Read the model definition and answer for the solid it produces. Units are mm, in the model's axes. Face numbers are marked on the shaded views. A direction names the side the tool comes from. Give positions to 0.01 mm unless a question says otherwise; leave off trailing zeros. Loops run counter-clockwise (first coordinate to the right, second up) from the corner with the lowest first, then second, coordinate; pieces in that order, holes last. Notation, with made-up numbers: (22.5, 25.25) -> (68.5, 25.25) arc R16 ccw to (68.5, 47.25) -> close; hole circle Ø5 at (-25, 10.5). An arc over 180 degrees is marked (long way). Return JSON: item names as keys, results as strings. Group by question number.
Autodesk Inventor part; units mm, degrees
ref_plane "YZ Plane" through (0, 0, 0) normal (1, 0, 0) x (0, 1, 0)
ref_plane "XZ Plane" through (0, 0, 0) normal (0, 1, 0) x (-1, 0, 0)
ref_plane "XY Plane" through (0, 0, 0) normal (0, 0, 1) x (1, 0, 0)
sketch "Sketch1" plane through (0, 0, 0) normal (0, 1, 0) x (-1, 0, 0)
  line L0 (41.275, 29.845) -> (-4.445, 29.845)
  line L1 (-4.445, 29.845) -> (-4.445, -10.795)
  line L2 (-4.445, -10.795) -> (41.275, -10.795)
  line L3 (41.275, -10.795) -> (41.275, 29.845)
  circle A0 centre (36.83, 19.05) radius 2.54
  circle A1 centre (36.83, 0) radius 2.54
  circle A2 centre (0, 0) radius 2.54
  circle A3 centre (0, 19.05) radius 2.54
  dimension "d1" = 19.05
  dimension "d2" = 36.83
  dimension "d20" = 40.64
  dimension "d21" = 45.72
  dimension "d22" = 10.795
  dimension "d23" = 4.445
  dimension "d24" = 19.05
  dimension "d25" = 10.795
  dimension "d26" = 36.83
  dimension "d27" = 4.445
  dimension "d28" = 4.445
  dimension "d31" = 5.08
  dimension "d32" = 5.08
  dimension "d33" = 5.08
  dimension "d34" = 5.08
extrude "Extrusion5" add sketch "Sketch1" along normal blind 40.64
sketch "Sketch4" plane through (0, 40.64, 0) normal (0, 1, 0) x (1, 0, 0)
  point P0 (0, 0)
  point P1 (-18.4878, -9.5896)
sketch "Sketch5" plane through (4.445, 0, 29.845) normal (1, 0, 0) x (0, 0, -1)
  line L0 (0, 40.64) -> (40.64, 0)
  line L1 (40.64, 40.64) -> (0, 0)
  circle A0 centre (20.32, 20.32) radius 7.62
  point P0 (29.845, 0)
  dimension "d38" = 15.24
extrude "Extrusion6" add sketch "Sketch5" along normal blind 40.64
sketch "Sketch6" plane through (-41.275, 0, -10.795) normal (-1, 0, 0) x (0, 0, 1)
  line L0 (0, 40.64) -> (40.64, 0)
  line L1 (40.64, 40.64) -> (0, 0)
  circle A0 centre (20.32, 20.32) radius 20.32
  point P0 (10.795, 0)
  dimension "d41" = 40.64
extrude "Extrusion7" add sketch "Sketch6" along normal blind 50.8
properties part number "P60 Gear Box"
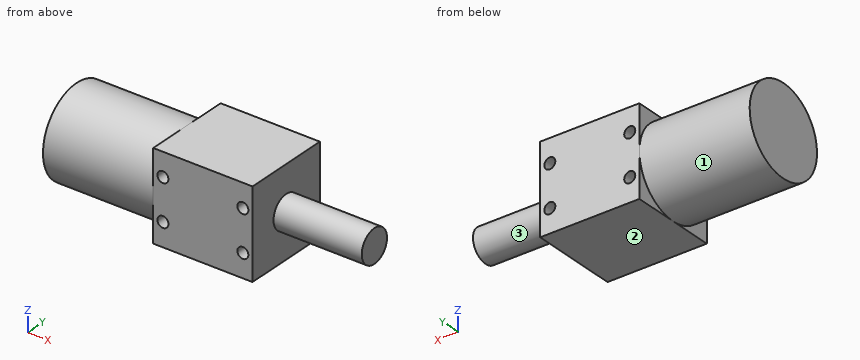
1. Section D-D on y = 23 is taken. State how many separate pieces and enclosed holes the cut face has, then the cut area to 3 significant figures.
2. Which of the six approach directions +Z, -Z, +X, -X, +Y, -Y give full straight-line access (tool end or side, diameter ignored) to the marked faces 1, 2 and 3?
3. Flat-ended cylindrical pins translate along their axes: pin 1 Ø6.5 at (x, z) = (0, 19.05) entering from +Y; pin 2 Ø3 at (x, y) = (-58, 32) entering from +Z; pin 3 Ø5 at (x, z) = (13.5, 11.5) entering from +Y; pin 4 Ø1.5 at (y, z) = (35, -3) entering from +X (3 decimals). Find the tip coordinate at first contact, or state that the pin passes through.
4. Straight lines are drawn through the part: line 1 (Z direction, x = 0, y = 17.5) (3 decimals); line 2 (X direction, y = 28, z = 19) (1 decimal); line 3 (Z direction, x = -36, y = 26) (3 decimals). For each, find the intervals that lie inside material, in ascending order. Write a range as from..to.
5. Section B-B on z = 19.05 is taken. Determine the outline of the cut face in (x, y) (3 decimals), then the cut area to 3 significant figures.
6. Section C-C on y = 33.5 is taken. Determine the outline of the cut face in (x, z) (3 decimals).
7. Section A-A on x = -36.83 is taken. Determine the outline of the cut face in (y, z) (3 decimals).
Completed:
{
 "1": {"separate pieces": "1", "enclosed holes": "4", "area": "4,400 mm²"},
 "2": {"face 1": "-X", "face 2": "-Z, +X, -X, +Y, -Y", "face 3": "+X"},
 "3": {"pin 1": "stops at y = 40.64", "pin 2": "stops at z = 27.11", "pin 3": "stops at y = 27.94", "pin 4": "stops at x = 4.445"},
 "4": {"line 1": "z = -10.795..-2.54, 2.54..16.51, 21.59..29.845", "line 2": "x = -92.1..-39.4, -34.3..-2.5, 2.5..4.4", "line 3": "z = -10.795..-2.401, 2.401..16.649, 21.451..29.845"},
 "5": {"outline": "(-92.075, 2.371) -> (-41.275, 2.371) -> (-41.275, 0) -> (-39.37, 0) -> (-39.37, 40.64) -> (-41.275, 40.64) -> (-41.275, 38.269) -> (-92.075, 38.269) -> close; (-34.29, 0) -> (-2.54, 0) -> (-2.54, 40.64) -> (-34.29, 40.64) -> close; (2.54, 0) -> (4.445, 0) -> (4.445, 40.64) -> (2.54, 40.64) -> close", "area": "3,270 mm²"},
 "6": {"outline": "(-92.075, -5.941) -> (-41.275, -5.941) -> (-41.275, -10.795) -> (4.445, -10.795) -> (4.445, 29.845) -> (-41.275, 29.845) -> (-41.275, 24.991) -> (-92.075, 24.991) -> close; hole circle Ø5.08 at (-36.83, 0); hole circle Ø5.08 at (-36.83, 19.05); hole circle Ø5.08 at (0, 0); hole circle Ø5.08 at (0, 19.05)"},
 "7": {"outline": "(0, -10.795) -> (40.64, -10.795) -> (40.64, -2.54) -> (0, -2.54) -> close; (0, 2.54) -> (40.64, 2.54) -> (40.64, 16.51) -> (0, 16.51) -> close; (0, 21.59) -> (40.64, 21.59) -> (40.64, 29.845) -> (0, 29.845) -> close"}
}
